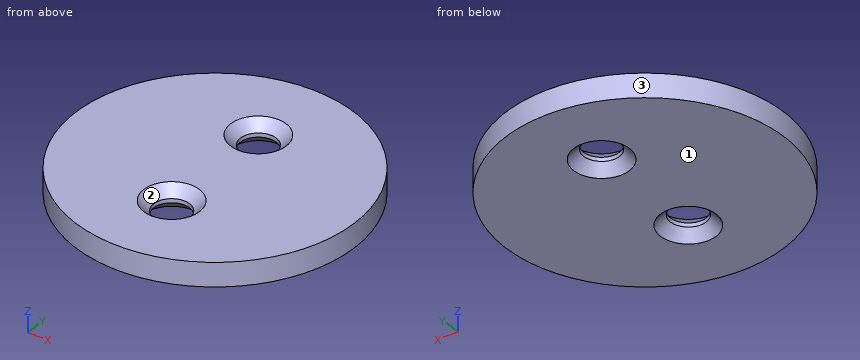
from build123d import *

# Parameters (mm, degrees)
SKETCH_1_R          = 7
EXTRUDE_1_DEPTH     = 1.2
SKETCH_2_R          = 0.9
CUT_EXTRUDE_1_DEPTH = 10.97196069
CHAMFER_1_SIZE      = 0.5


with BuildPart() as part:
    # 草图1 → 凸台-拉伸1 (new body)
    with BuildSketch(Plane.XY):
        Circle(SKETCH_1_R)
    extrude(amount=EXTRUDE_1_DEPTH)

    # 草图2 → 切除-拉伸1 (cut, through all)
    with BuildSketch(Plane.XY.offset(1.2)):
        with Locations((0, 3)):
            Circle(SKETCH_2_R)
        with Locations(Location((0, -3, 0), (0, 0, 180))):
            Circle(SKETCH_2_R)
    extrude(amount=-CUT_EXTRUDE_1_DEPTH, mode=Mode.SUBTRACT)

    # Chamfer 1
    chamfer_1_edges = [part.edges().sort_by_distance(p)[0] for p in [
        (0.9, -3, 1.2),
        (-0.9, 3, 0),
        (-0.9, 3, 1.2),
        (0.9, -3, 0),
    ]]
    chamfer(chamfer_1_edges, length=CHAMFER_1_SIZE)


solid = part.part
Design review of the part built by this model. Coordinates are the model's own, in mm. Face numbers are marked on the shaded views. Give positions to 0.01 mm unless a question says otherwise; leave off trailing zeros. Order: outer loops, then holes, each group sorted by start corner. A loop starts at its lowest first (then second) coordinate and runs counter-clockwise, first axis right, second up. Notation, with made-up numbers: (67, -30.5) - (91, -30.5) arc R18 cw to (91, -14.5) - close; hole circle Ø5 at (19, 69). An arc over 180 degrees is marked (long way). Write item = value, one per line. Start each with the question number.
Q1. We need section B-B on y = -3. State the section outline as (x, z) points.
Q2. We need section C-C on z = 1. State the section outline as (x, y) points, plus the area to 3 significant figures.
Q3. Clearance check with flat-ended pins moving along their axes: pin 1 Ø1.1 at (x, y) = (0, -3) entering from -Z; pin 2 Ø2.5 at (x, y) = (0, 3) entering from +Z. State where each tip first meets the part, or that it passes through.
Q4. We need section D-D on x = 2.5. State the section outline as (y, z) points.
Q5. We need section A-A on x = 0. State the section outline as (y, z) points, plus the area to 3 significant figures.
Q6. To check wall thickness, follow L1, parallel to Y at x = 0, z = 0.6; L2, parallel to Y at x = 1, z = 1.15; L3, parallel to X at y = 2.5, z = 1. State the ranges of each line that lie inside material, in increasing order. Write a range as from..to.
Q7. Mouldability with a two-part tool opening along X and no side actions: class the marked faces 1, 2 and 3 as released by +X, released by -X, zero draft, split by the parting line, or undercut.
Working result:
q1.outline = (-6.32, 0) - (-1.4, 0) - (-0.9, 0.5) - (-0.9, 0.7) - (-1.4, 1.2) - (-6.32, 1.2) - close; (0.9, 0.5) - (1.4, 0) - (6.32, 0) - (6.32, 1.2) - (1.4, 1.2) - (0.9, 0.7) - close
q2.outline = circle Ø14 at (0, 0); hole circle Ø2.4 at (0, -3); hole circle Ø2.4 at (0, 3)
q2.area = 145 mm²
q3.pin_1 = through
q3.pin_2 = 1.05
q4.outline = (-6.54, 0) - (6.54, 0) - (6.54, 1.2) - (-6.54, 1.2) - close
q5.outline = (-7, 0) - (-4.4, 0) - (-3.9, 0.5) - (-3.9, 0.7) - (-4.4, 1.2) - (-7, 1.2) - close; (-2.1, 0.5) - (-1.6, 0) - (1.6, 0) - (2.1, 0.5) - (2.1, 0.7) - (1.6, 1.2) - (-1.6, 1.2) - (-2.1, 0.7) - close; (3.9, 0.5) - (4.4, 0) - (7, 0) - (7, 1.2) - (4.4, 1.2) - (3.9, 0.7) - close
q5.area = 11.5 mm²
q6.L1 = -7..-3.9, -2.1..2.1, 3.9..7
q6.L2 = -6.93..-3.91, -2.09..2.09, 3.91..6.93
q6.L3 = -6.54..-1.09, 1.09..6.54
q7.face_1 = zero draft
q7.face_2 = undercut
q7.face_3 = split by the parting line
